```python
from build123d import *

# Parameters (mm, degrees)
F1_DEPTH = 12
F2_DEPTH = 16
F3_DEPTH = 25


with BuildPart() as f1:
    # F0 (on Top) → F1 (new body)
    with BuildSketch(Plane.XY):
        with BuildLine():
            ThreePointArc((-21.2132034356, 21.2132034356), (-16.3478362021, 25.1544877012), (-10.7703296143, 28))
            Line((-10.7703296143, 28), (-35.2278299076, 28))
            ThreePointArc((-35.2278299076, 28), (-45, 0), (-35.2278299076, -28))
            Line((-35.2278299076, -28), (-10.7703296143, -28))
            ThreePointArc((-10.7703296143, -28), (-16.3478362021, -25.1544877012), (-21.2132034356, -21.2132034356))
            ThreePointArc((-21.2132034356, -21.2132034356), (-30, 0), (-21.2132034356, 21.2132034356))
        make_face()
    extrude(amount=F1_DEPTH)



with BuildPart() as f1b:
    # F0 (on Top) → F1, piece 2 (new body)
    with BuildSketch(Plane.XY):
        with BuildLine():
            ThreePointArc((21.2132034356, 21.2132034356), (27.7163859753, 11.480502971), (30, 0))
            ThreePointArc((30, 0), (27.7163859753, -11.480502971), (21.2132034356, -21.2132034356))
            ThreePointArc((21.2132034356, -21.2132034356), (16.3478362021, -25.1544877012), (10.7703296143, -28))
            Line((10.7703296143, -28), (35.2278299076, -28))
            ThreePointArc((35.2278299076, -28), (45, 0), (35.2278299076, 28))
            Line((35.2278299076, 28), (10.7703296143, 28))
            ThreePointArc((10.7703296143, 28), (16.3478362021, 25.1544877012), (21.2132034356, 21.2132034356))
        make_face()
    extrude(amount=F1_DEPTH)


with BuildPart() as f1_1:
    add(f1.part)

    add(f1b.part)  # F2 merges F1b
    # F0 (on Top) → F2 (join)
    with BuildSketch(Plane.XY):
        with BuildLine():
            Line((10.6066017178, 10.6066017178), (21.2132034356, 21.2132034356))
            ThreePointArc((21.2132034356, 21.2132034356), (16.3478362021, 25.1544877012), (10.7703296143, 28))
            ThreePointArc((10.7703296143, 28), (0, 30), (-10.7703296143, 28))
            ThreePointArc((-10.7703296143, 28), (-16.3478362021, 25.1544877012), (-21.2132034356, 21.2132034356))
            Line((-21.2132034356, 21.2132034356), (-10.6066017178, 10.6066017178))
            ThreePointArc((-10.6066017178, 10.6066017178), (-15, 0), (-10.6066017178, -10.6066017178))
            Line((-10.6066017178, -10.6066017178), (-21.2132034356, -21.2132034356))
            ThreePointArc((-21.2132034356, -21.2132034356), (-16.3478362021, -25.1544877012), (-10.7703296143, -28))
            ThreePointArc((-10.7703296143, -28), (0, -30), (10.7703296143, -28))
            ThreePointArc((10.7703296143, -28), (16.3478362021, -25.1544877012), (21.2132034356, -21.2132034356))
            Line((21.2132034356, -21.2132034356), (10.6066017178, -10.6066017178))
            ThreePointArc((10.6066017178, -10.6066017178), (15, 0), (10.6066017178, 10.6066017178))
        make_face()
    extrude(amount=F2_DEPTH)

    # F0 (on Top) → F3 (join)
    with BuildSketch(Plane.XY):
        with BuildLine():
            ThreePointArc((21.2132034356, -21.2132034356), (27.7163859753, -11.480502971), (30, 0))
            ThreePointArc((30, 0), (27.7163859753, 11.480502971), (21.2132034356, 21.2132034356))
            Line((21.2132034356, 21.2132034356), (10.6066017178, 10.6066017178))
            ThreePointArc((10.6066017178, 10.6066017178), (15, 0), (10.6066017178, -10.6066017178))
            Line((10.6066017178, -10.6066017178), (21.2132034356, -21.2132034356))
        make_face()
        with BuildLine():
            Line((-10.6066017178, 10.6066017178), (-21.2132034356, 21.2132034356))
            ThreePointArc((-21.2132034356, 21.2132034356), (-30, 0), (-21.2132034356, -21.2132034356))
            Line((-21.2132034356, -21.2132034356), (-10.6066017178, -10.6066017178))
            ThreePointArc((-10.6066017178, -10.6066017178), (-15, 0), (-10.6066017178, 10.6066017178))
        make_face()
    extrude(amount=F3_DEPTH)


solid = f1_1.part
```
Input: part model. Units: mm. Frame: model coordinates. A direction names the side the tool comes from. Coordinates: 2 decimals unless noted, no trailing zeros. Loops run counter-clockwise (first coordinate to the right, second up) from the corner with the lowest first, then second, coordinate; pieces in that order, holes last. Notation, with made-up numbers: M -29.5,14 L 8.5,14 A18 ccw 8.5,34 Z; hole C 60.25,33 d6. An arc over 180 degrees is marked long. Use a Markdown table: item, result. Add a question column.
1) Draft query along X for faces 4 (the flat face through (0, 0, 16)), 5 (the cylindrical face through (-9.03, -28.61, 15.1)), 6 (the flat face through (-1, 0, 0)). Return one class per face: +X half, -X half, draft (parallel to the pull), parting line (faces both ways), or undercut.
2) Set-up query: faces 1 (the flat face through (31, 0, 12)), 2 (the flat face through (-16, -16, 20)), 3 (the cylindrical face through (-15, 0, 20)). Return all of +Z, -Z, +X, -X, +Y, -Y with unobstructed straight access to the full face (end or side cutting, diameter ignored); none if empty.
3) Section C-C, the plane z = 9.75. Return the cut outline in (x, y).
4) Section B-B, the plane y = 0. Return the cut outline in (x, z).
5) Pin query (flat end, axial travel): P1, Ø13, axis at x = -20.5, z = 3.5, coming from the +Y side; P2, Ø13, axis at x = 25, z = 3.5, coming from the -Y side; P3, Ø4, axis at x = -26.5, z = 19, coming from the +Y side; P4, Ø1, axis at x = 16.5, y = 2.5, coming from the -Z side. Return the tip coordinate at first contact, or that it passes through.
6) Section A-A, the plane x = 18. Return the cut outline in (y, z).
7) Line query: L1, parallel to Z at x = 0.5, y = 11; L2, parallel to Z at x = 38.5, y = -21; L3, parallel to X at y = 13, z = 23.25. Output: solid intervals per line, ascending. Write a range as from..to.
8) Section D-D, the plane x = -25.5. Return the cut outline in (y, z).
Answer below:
| question | item | result |
|---|---|---|
| 1 | face 4 | undercut |
| 1 | face 5 | parting line |
| 1 | face 6 | draft |
| 2 | face 1 | +Z, +X |
| 2 | face 2 | +Z, -Y |
| 2 | face 3 | +Z |
| 3 | outline | M -35.23,-28 L -10.77,-28 A30 ccw 10.77,-28 L 35.23,-28 A45 ccw 35.23,28 L 10.77,28 A30 ccw -10.77,28 L -35.23,28 A45 ccw Z |
| 4 | outline | M -45,0 L 45,0 L 45,12 L 30,12 L 30,25 L 15,25 L 15,16 L -15,16 L -15,25 L -30,25 L -30,12 L -45,12 Z |
| 5 | P1 | y = 28 |
| 5 | P2 | y = -28 |
| 5 | P3 | y = 17.31 |
| 5 | P4 | z = 0 |
| 6 | outline | M -28,0 L 28,0 L 28,12 L 24,12 L 24,16 L 18,16 L 18,25 L -18,25 L -18,16 L -24,16 L -24,12 L -28,12 Z |
| 7 | L1 | 0..16 |
| 7 | L2 | 0..12 |
| 7 | L3 | -27.04..-13, 13..27.04 |
| 8 | outline | M -28,0 L 28,0 L 28,12 L 15.8,12 L 15.8,25 L -15.8,25 L -15.8,12 L -28,12 Z |
